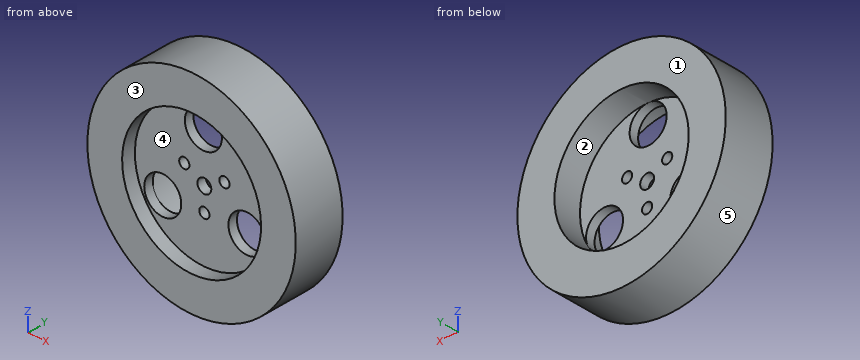
```python
from build123d import *

# Parameters (mm, degrees)
SKETCH1_R           = 22.5
BOSS_EXTRUDE1_DEPTH = 11
SKETCH2_R           = 14.5
CUT_EXTRUDE1_DEPTH  = 6
SKETCH3_R           = 15
CUT_EXTRUDE2_DEPTH  = 3
CUT_EXTRUDE3_REACH  = 34.381
SKETCH4_R           = 1.5
SKETCH4_R_2         = 1.1
SKETCH4_R_3         = 4


with BuildPart() as part:
    # Sketch1 → Boss-Extrude1 (new body)
    with BuildSketch(Plane(origin=(0, 0, 0), x_dir=(1, 0, 0), z_dir=(0, 1, 0))):
        with Locations(Location((0, 0, 0), (0, 0, 270))):
            Circle(SKETCH1_R)
    extrude(amount=BOSS_EXTRUDE1_DEPTH)

    # Sketch2 → Cut-Extrude1 (cut)
    with BuildSketch(Plane(origin=(0, 11, 0), x_dir=(1, 0, 0), z_dir=(0, 1, 0))):
        with Locations(Location((0, 0, 0), (0, 0, 270))):
            Circle(SKETCH2_R)
    extrude(amount=-CUT_EXTRUDE1_DEPTH, mode=Mode.SUBTRACT)

    # Sketch3 → Cut-Extrude2 (cut)
    with BuildSketch(Plane.XZ):
        with Locations(Location((0, 0, 0), (0, 0, 270))):
            Circle(SKETCH3_R)
    extrude(amount=-CUT_EXTRUDE2_DEPTH, mode=Mode.SUBTRACT)

    # Sketch4 → Cut-Extrude3 (cut, up to next)
    with BuildSketch(Plane(origin=(0, 5, 0), x_dir=(1, 0, 0), z_dir=(0, 1, 0)), mode=Mode.PRIVATE) as cut_extrude3_sk1:
        with Locations(Location((0, 0, 0), (0, 0, 270))):
            Circle(SKETCH4_R)
    cut_extrude3_tool1 = extrude(cut_extrude3_sk1.sketch, amount=-CUT_EXTRUDE3_REACH, mode=Mode.PRIVATE) & part.part
    # Sketch4 → Cut-Extrude3 (cut, up to next)
    with BuildSketch(Plane(origin=(0, 5, 0), x_dir=(1, 0, 0), z_dir=(0, 1, 0)), mode=Mode.PRIVATE) as cut_extrude3_sk2:
        with Locations(Location((0, 5, 0), (0, 0, 270))):
            Circle(SKETCH4_R_2)
    cut_extrude3_tool2 = extrude(cut_extrude3_sk2.sketch, amount=-CUT_EXTRUDE3_REACH, mode=Mode.PRIVATE) & part.part
    # Sketch4 → Cut-Extrude3 (cut, up to next)
    with BuildSketch(Plane(origin=(0, 5, 0), x_dir=(1, 0, 0), z_dir=(0, 1, 0)), mode=Mode.PRIVATE) as cut_extrude3_sk3:
        with Locations(Location((4.330127019, -2.5, 0), (0, 0, 270))):
            Circle(SKETCH4_R_2)
    cut_extrude3_tool3 = extrude(cut_extrude3_sk3.sketch, amount=-CUT_EXTRUDE3_REACH, mode=Mode.PRIVATE) & part.part
    # Sketch4 → Cut-Extrude3 (cut, up to next)
    with BuildSketch(Plane(origin=(0, 5, 0), x_dir=(1, 0, 0), z_dir=(0, 1, 0)), mode=Mode.PRIVATE) as cut_extrude3_sk4:
        with Locations(Location((-4.330127019, -2.5, 0), (0, 0, 270))):
            Circle(SKETCH4_R_2)
    cut_extrude3_tool4 = extrude(cut_extrude3_sk4.sketch, amount=-CUT_EXTRUDE3_REACH, mode=Mode.PRIVATE) & part.part
    # Sketch4 → Cut-Extrude3 (cut, up to next)
    with BuildSketch(Plane(origin=(0, 5, 0), x_dir=(1, 0, 0), z_dir=(0, 1, 0)), mode=Mode.PRIVATE) as cut_extrude3_sk5:
        with Locations(Location((9.198755892, 5.062893446, 0), (0, 0, 28.828375855))):
            Circle(SKETCH4_R_3)
    cut_extrude3_tool5 = extrude(cut_extrude3_sk5.sketch, amount=-CUT_EXTRUDE3_REACH, mode=Mode.PRIVATE) & part.part
    # Sketch4 → Cut-Extrude3 (cut, up to next)
    with BuildSketch(Plane(origin=(0, 5, 0), x_dir=(1, 0, 0), z_dir=(0, 1, 0)), mode=Mode.PRIVATE) as cut_extrude3_sk6:
        with Locations(Location((-0.214783605, -10.497803008, 0), (0, 0, 268.828376506))):
            Circle(SKETCH4_R_3)
    cut_extrude3_tool6 = extrude(cut_extrude3_sk6.sketch, amount=-CUT_EXTRUDE3_REACH, mode=Mode.PRIVATE) & part.part
    # Sketch4 → Cut-Extrude3 (cut, up to next)
    with BuildSketch(Plane(origin=(0, 5, 0), x_dir=(1, 0, 0), z_dir=(0, 1, 0)), mode=Mode.PRIVATE) as cut_extrude3_sk7:
        with Locations(Location((-8.983972287, 5.434909563, 0), (0, 0, 148.828375289))):
            Circle(SKETCH4_R_3)
    cut_extrude3_tool7 = extrude(cut_extrude3_sk7.sketch, amount=-CUT_EXTRUDE3_REACH, mode=Mode.PRIVATE) & part.part
    add(cut_extrude3_tool1.solids().sort_by_distance((0, 5, 0))[0], mode=Mode.SUBTRACT)
    add(cut_extrude3_tool2.solids().sort_by_distance((0, 5, -5))[0], mode=Mode.SUBTRACT)
    add(cut_extrude3_tool3.solids().sort_by_distance((4.330127, 5, 2.5))[0], mode=Mode.SUBTRACT)
    add(cut_extrude3_tool4.solids().sort_by_distance((-4.330127, 5, 2.5))[0], mode=Mode.SUBTRACT)
    add(cut_extrude3_tool5.solids().sort_by_distance((9.198756, 5, -5.062893))[0], mode=Mode.SUBTRACT)
    add(cut_extrude3_tool6.solids().sort_by_distance((-0.214784, 5, 10.497803))[0], mode=Mode.SUBTRACT)
    add(cut_extrude3_tool7.solids().sort_by_distance((-8.983972, 5, -5.43491))[0], mode=Mode.SUBTRACT)


solid = part.part
```
Check sheet for the modelled part. Datum: model origin and axes. Units: mm. Face numbers are marked on the shaded views. A direction names the side the tool comes from. Round coordinates to 2 decimals unless told otherwise and drop trailing zeros. Loops run counter-clockwise (first coordinate to the right, second up) from the corner with the lowest first, then second, coordinate; pieces in that order, holes last. Notation, with made-up numbers: (39.5, 62.25) - (48.5, 62.25) arc R12 ccw to (48.5, 72.25) - close; hole circle Ø9 at (81, 46.5). An arc over 180 degrees is marked (long way). Answer as a JSON object with one key per item and string values. Group by question number.
Q1. Mould release check, pull along X, two halves, no side actions. Record for the marked faces 3, 4 and 5: released by +X, released by -X, zero draft, split by the parting line, or undercut.
Q2. Sectioned sample at A-A, the plane z = 0. Enter the section's corners in (x, y).
Q3. Set-up check for the marked faces 1 and 2: record each of +Z, -Z, +X, -X, +Y, -Y from which the full face is reachable in a straight line by a thin tool's end or side.
Q4. Sectioned sample at C-C, the plane y = 3.75. Enter the section's corners in (x, z).
Q5. Scan lines: line 1 along X through (y, z) = (1.95, 0); line 2 along X through (y, z) = (4.25, -2); line 3 along Y through (x, z) = (-2, 0.5). Record each from-to range of solid material in increasing order. Write a range as [from, to].
Q6. Sectioned sample at B-B, the plane x = 8.5. Enter the section's corners in (y, z).
Q7. Gauge pin test, flat ends, axial feed: P1, Ø3, axis at y = 9, z = -11, coming from the +X side; P2, Ø3.5, axis at x = 0, z = -5, coming from the -Y side; P3, Ø5, axis at x = 0, z = 0, coming from the +Y side. Record the tip position at first contact, or that the pin passes through.
Solution:
{
 "1": {"face 3": "zero draft", "face 4": "undercut", "face 5": "split by the parting line"},
 "2": {"outline": "(-22.5, 0) - (-15, 0) - (-15, 3) - (-1.5, 3) - (-1.5, 5) - (-14.5, 5) - (-14.5, 11) - (-22.5, 11) - close; (1.5, 3) - (15, 3) - (15, 0) - (22.5, 0) - (22.5, 11) - (14.5, 11) - (14.5, 5) - (1.5, 5) - close"},
 "3": {"face 1": "+Z, -Z, +X, -X, +Y", "face 2": "+Y"},
 "4": {"outline": "circle Ø45 at (0, 0); hole circle Ø8 at (-8.98, -5.43); hole circle Ø2.2 at (-4.33, 2.5); hole circle Ø8 at (-0.21, 10.5); hole circle Ø3 at (0, 0); hole circle Ø2.2 at (0, -5); hole circle Ø2.2 at (4.33, 2.5); hole circle Ø8 at (9.2, -5.06)"},
 "5": {"line 1": "x = [-22.5, -15], [15, 22.5]", "line 2": "x = [-22.41, -11.03], [-6.93, 6.63], [11.77, 22.41]", "line 3": "y = [3, 5]"},
 "6": {"outline": "(0, -20.83) - (11, -20.83) - (11, -11.75) - (5, -11.75) - (5, -9) - (3, -9) - (3, -12.36) - (0, -12.36) - close; (0, 12.36) - (3, 12.36) - (3, -1.12) - (5, -1.12) - (5, 11.75) - (11, 11.75) - (11, 20.83) - (0, 20.83) - close"},
 "7": {"P1": "stops at x = 20.4", "P2": "stops at y = 3", "P3": "stops at y = 5"}
}
